For this review, take the finished solid that the model builds, in its own axes (mm). Round coordinates to 2 decimals unless told otherwise and drop trailing zeros. Loops run counter-clockwise (first coordinate to the right, second up) from the corner with the lowest first, then second, coordinate; pieces in that order, holes last.
1. Clearance check with flat-ended pins moving along their axes: pin 1 Ø0.8 at (x, y) = (-187, 1) entering from +Z; pin 2 Ø1.4 at (y, z) = (1.5, -1.5) entering from +X; pin 3 Ø2 at (x, z) = (-36, 57) entering from -Y; pin 4 Ø0.8 at (y, z) = (1, -1.5) entering from -X. State where each tip first meets the part, or that it passes through.
2. Consider section A-A on y = 0.8. State the section outline as (x, z) points.
3. To check wall thickness, follow line 1 along Z through (x, y) = (-126.5, 2.65). State the ranges of the line that lie inside material, in increasing order.
4. Consider section B-B on x = -68.5. State the section outline as (y, z) points.
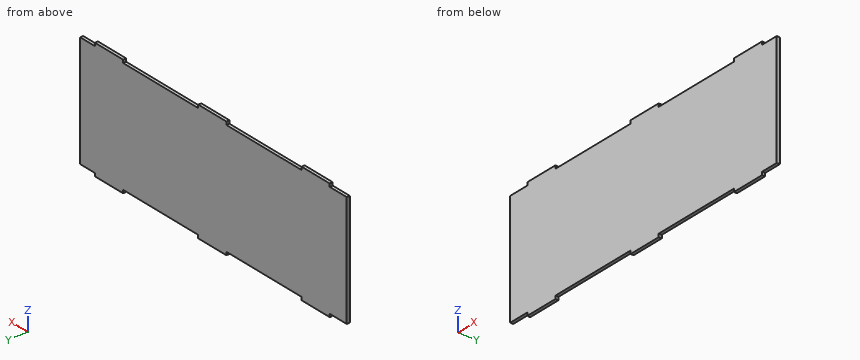
from build123d import *

# Parameters (mm, degrees)
SKETCH1_W           = 300
SKETCH1_H           = 2.7
BOSS_EXTRUDE1_DEPTH = 100
SKETCH3_W           = 30
SKETCH3_H           = 2.7
BOSS_EXTRUDE2_DEPTH = 2.7
SKETCH4_W           = 11.849818602
SKETCH4_H           = 2.7
CUT_EXTRUDE1_DEPTH  = 318.103421615
SKETCH5_W           = 4.361423596
SKETCH5_H           = 100
CUT_EXTRUDE2_DEPTH  = 2.7


with BuildPart() as part:
    # Sketch1 → Boss-Extrude1 (new body)
    with BuildSketch(Plane.XY):
        with Locations((-150, 1.35)):
            Rectangle(SKETCH1_W, SKETCH1_H)
    extrude(amount=BOSS_EXTRUDE1_DEPTH)

    # Sketch3 → Boss-Extrude2 (add)
    with BuildSketch(Plane(origin=(0, 2.7, 0), x_dir=(1, 0, 0), z_dir=(0, 1, 0))):
        with Locations((-35, 1.35)):
            Rectangle(SKETCH3_W, SKETCH3_H)
        with Locations((-145, 1.35)):
            Rectangle(SKETCH3_W, SKETCH3_H)
        with Locations((-255, 1.35)):
            Rectangle(SKETCH3_W, SKETCH3_H)
        with Locations((-255, -101.35)):
            Rectangle(SKETCH3_W, SKETCH3_H)
        with Locations((-145, -101.35)):
            Rectangle(SKETCH3_W, SKETCH3_H)
        with Locations((-35, -101.35)):
            Rectangle(SKETCH3_W, SKETCH3_H)
    extrude(amount=-BOSS_EXTRUDE2_DEPTH)

    # Sketch4 → Cut-Extrude1 (cut, through all)
    with BuildSketch(Plane(origin=(0, 0, 0), x_dir=(-1, 0, 0), z_dir=(0, 0, -1))):
        with Locations((294.075090699, 1.35)):
            Rectangle(SKETCH4_W, SKETCH4_H)
    extrude(amount=-CUT_EXTRUDE1_DEPTH, mode=Mode.SUBTRACT)

    # Sketch5 → Cut-Extrude2 (cut)
    with BuildSketch(Plane(origin=(0, 2.7, 0), x_dir=(1, 0, 0), z_dir=(0, 1, 0))):
        with Locations((-2.180711798, -50)):
            Rectangle(SKETCH5_W, SKETCH5_H)
    extrude(amount=-CUT_EXTRUDE2_DEPTH, mode=Mode.SUBTRACT)


solid = part.part
Resolved:
1. pin 1: stops at z = 100
1. pin 2: stops at x = -20
1. pin 3: stops at y = 0
1. pin 4: stops at x = -270
2. outline: (-288.15, 0) - (-270, 0) - (-270, -2.7) - (-240, -2.7) - (-240, 0) - (-160, 0) - (-160, -2.7) - (-130, -2.7) - (-130, 0) - (-50, 0) - (-50, -2.7) - (-20, -2.7) - (-20, 0) - (-4.36, 0) - (-4.36, 100) - (-20, 100) - (-20, 102.7) - (-50, 102.7) - (-50, 100) - (-130, 100) - (-130, 102.7) - (-160, 102.7) - (-160, 100) - (-240, 100) - (-240, 102.7) - (-270, 102.7) - (-270, 100) - (-288.15, 100) - close
3. line 1: z = 0 to 100
4. outline: (0, 0) - (2.7, 0) - (2.7, 100) - (0, 100) - close
